Work out the finished part from the listing and answer in its coordinate system (mm). Face numbers are marked on the shaded views. A direction names the side the tool comes from. Round coordinates to 2 decimals unless told otherwise and drop trailing zeros. Write each loop counter-clockwise with the first axis right and the second up, starting at its lowest first coordinate (ties: lowest second). Pieces come first, ordered by that corner, then holes. Notation, with made-up numbers: (35.5, 9.5) -> (66.5, 9.5) arc R23 cw to (66.5, 43.5) -> close; hole circle Ø4 at (34.5, -7.75). An arc over 180 degrees is marked (long way). One line per item, written item: value.
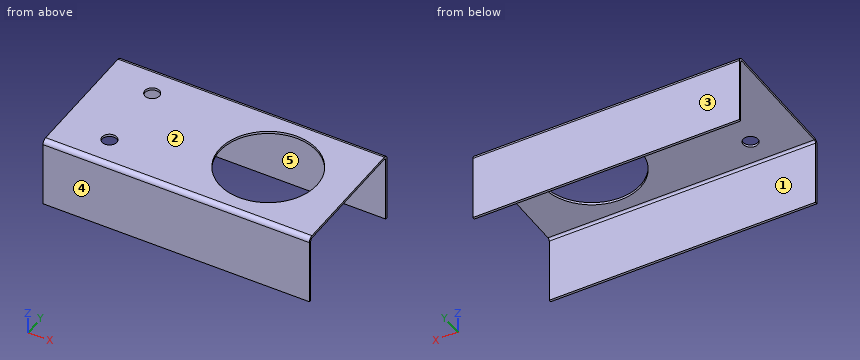
```python
from build123d import *

# Parameters (mm, degrees)
SKETCH1_W                    = 90
SKETCH1_H                    = 45.05
BASE_FLANGE1_DEPTH           = 0.81
EDGE_FLANGE1_STRIP_W         = 4.7132
EDGE_FLANGE1_STRIP_H         = 0.81
EDGE_FLANGE1_STRIP_CUT_DEPTH = 90
EDGE_FLANGE1_DEPTH           = 90
EDGE_FLANGE2_STRIP_W         = 4.7132
EDGE_FLANGE2_STRIP_H         = 0.81
EDGE_FLANGE2_STRIP_CUT_DEPTH = 90
EDGE_FLANGE2_DEPTH           = 90
SKETCH9_R                    = 16.5
SKETCH9_R_2                  = 2.5
CUT_EXTRUDE1_DEPTH           = 10


# Sheet-metal steps are written as plain solids
with BuildPart() as part:
    # Sketch1 → Base-Flange1 (new body)
    with BuildSketch(Plane.XY):
        with Locations((45, 22.525)):
            Rectangle(SKETCH1_W, SKETCH1_H)
    extrude(amount=-BASE_FLANGE1_DEPTH)

    # Edge-Flange1 strip (across the edge) → Edge-Flange1 strip cut (cut)
    with BuildSketch(Plane(origin=(0, 45.05, -0.81), x_dir=(0, -1, 0), z_dir=(1, 0, 0))):
        with Locations((-0.81, -0.405)):
            Rectangle(EDGE_FLANGE1_STRIP_W, EDGE_FLANGE1_STRIP_H)
    extrude(amount=EDGE_FLANGE1_STRIP_CUT_DEPTH, mode=Mode.SUBTRACT)

    # Edge-Flange1 section (across the edge) → Edge-Flange1 (add)
    with BuildSketch(Plane(origin=(0, 45.05, -0.81), x_dir=(0, -1, 0), z_dir=(1, 0, 0))):
        with BuildLine():
            Line((0, 0.7366), (0, 23))
            Line((0, 23), (0.81, 23))
            Line((0.81, 23), (0.81, 0.7366))
            ThreePointArc((0.81, 0.7366), (1.025745145, 0.215745145), (1.5466, 0))
            Line((1.5466, 0), (1.5466, -0.81))
            ThreePointArc((1.5466, -0.81), (0.452988652, -0.357011348), (0, 0.7366))
        make_face()
    extrude(amount=EDGE_FLANGE1_DEPTH)

    # Edge-Flange2 strip (across the edge) → Edge-Flange2 strip cut (cut)
    with BuildSketch(Plane(origin=(90, 0, -0.81), x_dir=(0, 1, 0), z_dir=(-1, 0, 0))):
        with Locations((-0.81, -0.405)):
            Rectangle(EDGE_FLANGE2_STRIP_W, EDGE_FLANGE2_STRIP_H)
    extrude(amount=EDGE_FLANGE2_STRIP_CUT_DEPTH, mode=Mode.SUBTRACT)

    # Edge-Flange2 section (across the edge) → Edge-Flange2 (add)
    with BuildSketch(Plane(origin=(90, 0, -0.81), x_dir=(0, 1, 0), z_dir=(-1, 0, 0))):
        with BuildLine():
            Line((0, 0.7366), (0, 23))
            Line((0, 23), (0.81, 23))
            Line((0.81, 23), (0.81, 0.7366))
            ThreePointArc((0.81, 0.7366), (1.025745145, 0.215745145), (1.5466, 0))
            Line((1.5466, 0), (1.5466, -0.81))
            ThreePointArc((1.5466, -0.81), (0.452988652, -0.357011348), (0, 0.7366))
        make_face()
    extrude(amount=EDGE_FLANGE2_DEPTH)

    # Sketch9 → Cut-Extrude1 (cut)
    with BuildSketch(Plane.XY):
        with Locations((63, 22.525)):
            Circle(SKETCH9_R)
        with Locations((16.55327865, 10.12)):
            Circle(SKETCH9_R_2)
        with Locations((16.55327865, 34.93)):
            Circle(SKETCH9_R_2)
    extrude(amount=-CUT_EXTRUDE1_DEPTH, mode=Mode.SUBTRACT)


solid = part.part
```
(1) Find section A-A on z = -19. Give the vertices of the cut face in (x, y).
Reported:
outline: (0, 0) -> (90, 0) -> (90, 0.81) -> (0, 0.81) -> close; (0, 44.24) -> (90, 44.24) -> (90, 45.05) -> (0, 45.05) -> close
(2) A flat-ended cylindrical pin translates along its axis: pin 1 Ø21 at (x, y) = (57.5, 31) entering from -Z. Find the tip coordinate at first contact, or state that the pin passes through.
Reported:
pin 1: stops at z = -0.81
(3) Find section B-B on x = 63. Give the vertices of the cut face in (y, z) (3 decimals), plus the area to 3 significant figures.
Reported:
outline: (0, -23.81) -> (0.81, -23.81) -> (0.81, -1.547) arc R0.737 cw to (1.547, -0.81) -> (6.025, -0.81) -> (6.025, 0) -> (1.547, 0) arc R1.547 ccw to (0, -1.547) -> close; (39.025, -0.81) -> (43.503, -0.81) arc R0.737 cw to (44.24, -1.547) -> (44.24, -23.81) -> (45.05, -23.81) -> (45.05, -1.547) arc R1.547 ccw to (43.503, 0) -> (39.025, 0) -> close
area: 46.2 mm2
(4) A tool of negligible diameter and unlimited length cuts with its end or side. For the marked faces 1 and 2, from which of +Z, -Z, +X, -X, +Y, -Y can it reach the whole face along a straight path? Write none if from no direction.
Reported:
face 1: -Z, +X, -X
face 2: +Z, +X, -X, +Y, -Y
(5) Consider probe 1 along Y at (x, z) = (75, -14.5); probe 2 along Z at (x, y) = (55.5, 3.5); probe 3 along Y at (x, z) = (82, -1.25). Determine where each line is inside the solid, lowest interval first.
Reported:
probe 1: y = 0 to 0.81, 44.24 to 45.05
probe 2: z = -0.81 to 0
probe 3: y = 0.03 to 0.87, 44.18 to 45.02
(6) For a pull along Y with two mould halves and no side action, classify the marked faces 3, 4 and 5 as pulls with the +Y half, pulls with the -Y half, needs draft (parallel to the pull), parting line crosses it, or undercut.
Reported:
face 3: pulls with the +Y half
face 4: pulls with the -Y half
face 5: undercut
(7) Find section C-C on x = 16. Give the vertices of the cut face in (y, z).
Reported:
outline: (0, -23.81) -> (0.81, -23.81) -> (0.81, -1.55) arc R0.74 cw to (1.55, -0.81) -> (7.68, -0.81) -> (7.68, 0) -> (1.55, 0) arc R1.55 ccw to (0, -1.55) -> close; (12.56, -0.81) -> (32.49, -0.81) -> (32.49, 0) -> (12.56, 0) -> close; (37.37, -0.81) -> (43.5, -0.81) arc R0.74 cw to (44.24, -1.55) -> (44.24, -23.81) -> (45.05, -23.81) -> (45.05, -1.55) arc R1.55 ccw to (43.5, 0) -> (37.37, 0) -> close
(8) Find section D-D on y = 28.5. Give the vertices of the cut face in (x, z), plus the area to 3 significant figures.
Reported:
outline: (0, -0.81) -> (47.62, -0.81) -> (47.62, 0) -> (0, 0) -> close; (78.38, -0.81) -> (90, -0.81) -> (90, 0) -> (78.38, 0) -> close
area: 48.0 mm2
